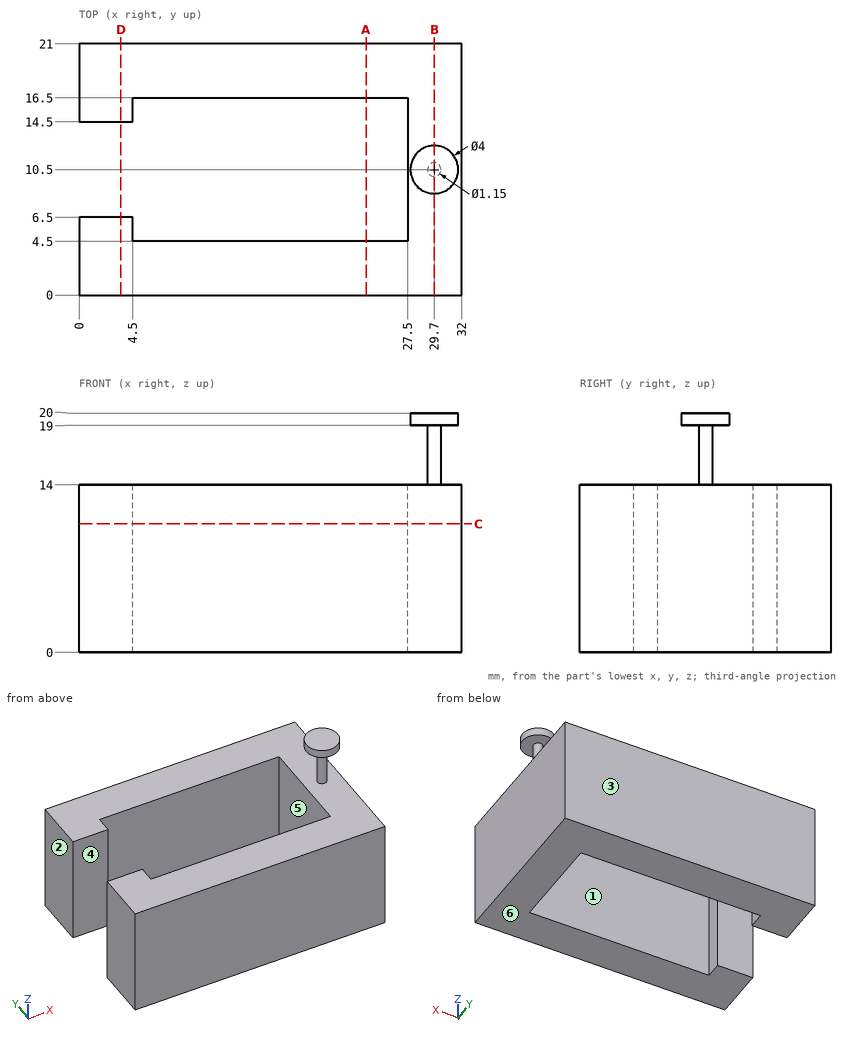
Can you work these out from the drawing? Everything is in mm from the part's minimum corner. A direction names the side the tool comes from. Coordinates: 2 decimals unless noted, no trailing zeros. Loops run counter-clockwise (first coordinate to the right, second up) from the corner with the lowest first, then second, coordinate; pieces in that order, holes last.
1. For P1, Ø4, axis at y = 2.5, z = 13.5, coming from the -X side; P2, Ø3.5, axis at y = 10.5, z = 7, coming from the -X side; P3, Ø4, axis at x = 5.5, y = 15.5, coming from the +Z side; P4, Ø1, axis at x = 14, z = 15.5, coming from the -Y side, each with a flat end and sliding along its axis, tell me the tip position at first contact or that it passes through.
2. I need wall thicknesses on L1, parallel to Y at x = 9, z = 11.25; L2, parallel to Y at x = 4, z = 3.75; L3, parallel to X at y = 15, z = 9. Which ranges of each line are inside material? Lowest first, please.
3. Imagine slicing it at A-A, the plane x = 24. Please give me the cut outline in (y, z).
4. For the marked faces 4, 5 and 6, which set-ups out of +Z, -Z, +X, -X, +Y, -Y let a thin tool reach every point of the face, with its end or its side?
5. Imagine slicing it at C-C, the plane z = 10.75. Please give me the cut outline in (x, y).
6. If we mould it in two halves opening along Y, with no side actions, what happens to the marked faces 1, 2 and 3? For each: pulls with the +Y half, pulls with the -Y half, needs draft (parallel to the pull), parting line crosses it, or undercut.
7. Imagine slicing it at B-B, the plane x = 29.7. Please give me the cut outline in (y, z) (3 decimals).
8. Imagine slicing it at D-D, the plane x = 3.5. Please give me the cut outline in (y, z).
Taken from the geometry:
1. P1: stops at x = 0
1. P2: stops at x = 27.5
1. P3: stops at z = 14
1. P4: passes through
2. L1: y = 0 to 4.5, 16.5 to 21
2. L2: y = 0 to 6.5, 14.5 to 21
2. L3: x = 0 to 4.5, 27.5 to 32
3. outline: (0, 0) - (4.5, 0) - (4.5, 14) - (0, 14) - close; (16.5, 0) - (21, 0) - (21, 14) - (16.5, 14) - close
4. face 4: +Z, -Z, -X
4. face 5: +Z, -Z
4. face 6: -Z, +X, -X, +Y, -Y
5. outline: (0, 0) - (32, 0) - (32, 21) - (0, 21) - (0, 14.5) - (4.5, 14.5) - (4.5, 16.5) - (27.5, 16.5) - (27.5, 4.5) - (4.5, 4.5) - (4.5, 6.5) - (0, 6.5) - close
6. face 1: undercut
6. face 2: needs draft
6. face 3: pulls with the +Y half
7. outline: (0, 0) - (21, 0) - (21, 14) - (11.075, 14) - (11.075, 19) - (12.5, 19) - (12.5, 20) - (8.5, 20) - (8.5, 19) - (9.925, 19) - (9.925, 14) - (0, 14) - close
8. outline: (0, 0) - (6.5, 0) - (6.5, 14) - (0, 14) - close; (14.5, 0) - (21, 0) - (21, 14) - (14.5, 14) - close
